```python
from build123d import *

# Parameters (mm, degrees)
SKETCH2_W                                      = 38.1
SKETCH2_H                                      = 6.35
BOSS_EXTRUDE2_DEPTH                            = 7.9375
CBORE_FOR_4_SOCKET_HEAD_CAP_SCREW1_D           = 3.2639
CBORE_FOR_4_SOCKET_HEAD_CAP_SCREW1_CBORE_D     = 5.55752
CBORE_FOR_4_SOCKET_HEAD_CAP_SCREW1_CBORE_DEPTH = 2.8448
CUT_EXTRUDE1_DEPTH                             = 12.7


with BuildPart() as part:
    # Sketch2 → Boss-Extrude2 (new body)
    with BuildSketch(Plane(origin=(0, 0, 0), x_dir=(1, 0, 0), z_dir=(0, 1, 0))):
        with Locations((19.05, 3.175)):
            Rectangle(SKETCH2_W, SKETCH2_H)
    extrude(amount=BOSS_EXTRUDE2_DEPTH)

    # CBORE for #4 Socket Head Cap Screw1 (through all)
    with Locations(Plane(origin=(6.35, 3.96875, 0), x_dir=(1, 0, 0), z_dir=(0, 0, 1))):
        with Locations((0, 0), (25.4, 0)):
            CounterBoreHole(CBORE_FOR_4_SOCKET_HEAD_CAP_SCREW1_D / 2, CBORE_FOR_4_SOCKET_HEAD_CAP_SCREW1_CBORE_D / 2, CBORE_FOR_4_SOCKET_HEAD_CAP_SCREW1_CBORE_DEPTH)

    # Sketch4 → Cut-Extrude1 (cut)
    with BuildSketch(Plane(origin=(0, 7.9375, 0), x_dir=(1, 0, 0), z_dir=(0, 1, 0))):
        Polygon((0, 0), (0, 2.54), (7.62, 0), align=None)
        Polygon((38.1, 2.54), (30.48, 0), (38.1, 0), align=None)
    extrude(amount=-CUT_EXTRUDE1_DEPTH, mode=Mode.SUBTRACT)


solid = part.part
```
Check sheet for the modelled part. Datum: model origin and axes. Units: mm. A direction names the side the tool comes from. Coordinates: 2 decimals unless noted, no trailing zeros. Order: outer loops, then holes, each group sorted by start corner. A loop starts at its lowest first (then second) coordinate and runs counter-clockwise, first axis right, second up. Notation, with made-up numbers: M 53,9 L 107,9 A13 ccw 107,19 Z; hole C 62.5,-12 d6. An arc over 180 degrees is marked long. Write each question's results on one line, items separated by ' | '. Start each with the question number.
1. Mould release check, pull along X, two halves, no side actions. Record for faces 3 (the face through (19, 0, -3)), 4 (the face through (28.974, 4.091, -1.719)), 5 (the face through (0, 4, -4)), 6 (the face through (8.917, 2.904, -1.719)): +X half, -X half, draft (parallel to the pull), parting line (faces both ways), or undercut.
2. Cross-section at C-C on z = -5.25. Record the cut outline in (x, y), and give its area (3 significant figures).
3. Go/stop test with a flat-tipped pin: P1, Ø4.5, axis at x = 6.35, y = 3.97, coming from the +Z side. Record where the tip stops, or that it passes through.
4. Material ranges on probe 1 along Y at (x, z) = (6.35, -4.9); probe 2 along Z at (x, y) = (8, 4.5); probe 3 along X at (y, z) = (4.25, -5.25), recorded low to high.
5. Cross-section at D-D on x = 8.5. Record the cut outline in (y, z), and give its area (3 significant figures).
6. Access from +Z, -Z, +X, -X, +Y, -Y to the whole of each face (thin tool, end or side, straight path). Record for faces 1 (the face through (38.1, 4, -4)), 2 (the face through (8, 3, -2.845)).
7. Cross-section at A-A on x = 33. Record the cut outline in (y, z).
8. Cross-section at B-B on y = 3.25. Record the cut outline in (x, z), and give its area (3 significant figures).
Checks:
1) face 3: draft | face 4: undercut | face 5: -X half | face 6: undercut
2) outline: M 0,0 L 38.1,0 L 38.1,7.94 L 0,7.94 Z; hole C 6.35,3.97 d3.26; hole C 31.75,3.97 d3.26 | area: 286 mm²
3) P1: stops at z = -2.84
4) probe 1: y = 0 to 2.34, 5.6 to 7.94 | probe 2: z = -6.35 to -2.84 | probe 3: x = 0 to 4.74, 7.96 to 30.14, 33.36 to 38.1
5) outline: M 0,-6.35 L 7.94,-6.35 L 7.94,0 L 5.73,0 L 5.73,-2.84 L 2.21,-2.84 L 2.21,0 L 0,0 Z | area: 40.4 mm²
6) face 1: +Z, -Z, +X, +Y, -Y | face 2: +Z
7) outline: M 0,-6.35 L 2.92,-6.35 L 2.92,-2.84 L 1.49,-2.84 L 1.49,-0.84 L 0,-0.84 Z; M 5.02,-6.35 L 7.94,-6.35 L 7.94,-0.84 L 6.45,-0.84 L 6.45,-2.84 L 5.02,-2.84 Z
8) outline: M 0,-6.35 L 4.88,-6.35 L 4.88,-2.84 L 3.67,-2.84 L 3.67,-1.32 L 0,-2.54 Z; M 7.82,-6.35 L 30.28,-6.35 L 30.28,-2.84 L 29.07,-2.84 L 29.07,0 L 9.03,0 L 9.03,-2.84 L 7.82,-2.84 Z; M 33.22,-6.35 L 38.1,-6.35 L 38.1,-2.54 L 34.43,-1.32 L 34.43,-2.84 L 33.22,-2.84 Z | area: 177 mm²
